from build123d import *

# Parameters (mm, degrees)
BOSS_EXTRUDE1_DEPTH = 18
SKETCH2_R           = 10
CUT_EXTRUDE1_DEPTH  = 5.6
SKETCH3_R           = 8.371578903
SKETCH3_R_2         = 6.7
BOSS_EXTRUDE2_DEPTH = 6.63


with BuildPart() as part:
    # Sketch1 → Boss-Extrude1 (new body)
    with BuildSketch(Plane.XY):
        with BuildLine():
            Line((15, 0), (75, 0))
            ThreePointArc((75, 0), (90, 15), (75, 30))
            Line((75, 30), (15, 30))
            ThreePointArc((15, 30), (0, 15), (15, 0))
        make_face()
        Polygon((15, 23.371578903), (7.75, 19.185789452), (7.75, 10.814210548), (15, 6.628421097), (22.25, 10.814210548), (22.25, 19.185789452), align=None, mode=Mode.SUBTRACT)
        Polygon((75, 23.371578903), (67.75, 19.185789452), (67.75, 10.814210548), (75, 6.628421097), (82.25, 10.814210548), (82.25, 19.185789452), align=None, mode=Mode.SUBTRACT)
    extrude(amount=BOSS_EXTRUDE1_DEPTH)

    # Sketch2 → Cut-Extrude1 (cut)
    with BuildSketch(Plane(origin=(0, 0, 0), x_dir=(-1, 0, 0), z_dir=(0, 0, -1))):
        with Locations((-75, 15)):
            Circle(SKETCH2_R)
        with Locations((-15, 15)):
            Circle(SKETCH2_R)
    extrude(amount=-CUT_EXTRUDE1_DEPTH, mode=Mode.SUBTRACT)

    # Sketch3 → Boss-Extrude2 (add)
    # profile 1 of 2: a face of its own
    with BuildSketch(Plane.XY.offset(18)):
        with Locations((75, 15)):
            Circle(SKETCH3_R)
        with Locations((75, 15)):
            Circle(SKETCH3_R_2, mode=Mode.SUBTRACT)
    # profile 2 of 2: a face of its own
    with BuildSketch(Plane.XY.offset(18)):
        with Locations((15, 15)):
            Circle(SKETCH3_R)
        with Locations((15, 15)):
            Circle(SKETCH3_R_2, mode=Mode.SUBTRACT)
    extrude(amount=-BOSS_EXTRUDE2_DEPTH)


solid = part.part
Build history of the part. All positions in model axes, mm. A direction names the side the tool comes from. Round coordinates to 2 decimals unless told otherwise and drop trailing zeros. Write each loop counter-clockwise with the first axis right and the second up, starting at its lowest first coordinate (ties: lowest second). Pieces come first, ordered by that corner, then holes. Notation, with made-up numbers: (10.5, -35.5) - (24.5, -35.5) arc R15 cw to (24.5, -6.5) - close; hole circle Ø3 at (-5.75, 55.5). An arc over 180 degrees is marked (long way). One line per question, with ' | ' between items.
1. Band-saw the part on A-A, the plane z = 7.75. Write the cut outline in (x, y), and give its area (3 significant figures).
Results are:
outline: (15, 0) - (75, 0) arc R15 ccw to (75, 30) - (15, 30) arc R15 ccw to start; hole (7.75, 10.81) - (15, 6.63) - (22.25, 10.81) - (22.25, 19.19) - (15, 23.37) - (7.75, 19.19) - close; hole (67.75, 10.81) - (75, 6.63) - (82.25, 10.81) - (82.25, 19.19) - (75, 23.37) - (67.75, 19.19) - close | area: 2,140 mm^2
2. Band-saw the part on C-C, the plane y = 20. Write the cut outline in (x, z).
Results are:
outline: (0.86, 0) - (6.34, 0) - (6.34, 5.6) - (9.16, 5.6) - (9.16, 11.37) - (10.54, 11.37) - (10.54, 18) - (0.86, 18) - close; (19.46, 11.37) - (20.84, 11.37) - (20.84, 5.6) - (23.66, 5.6) - (23.66, 0) - (66.34, 0) - (66.34, 5.6) - (69.16, 5.6) - (69.16, 11.37) - (70.54, 11.37) - (70.54, 18) - (19.46, 18) - close; (79.46, 11.37) - (80.84, 11.37) - (80.84, 5.6) - (83.66, 5.6) - (83.66, 0) - (89.14, 0) - (89.14, 18) - (79.46, 18) - close
3. Band-saw the part on D-D, the plane y = 12. Write the cut outline in (x, z), and give its area (3 significant figures).
Results are:
outline: (0.3, 0) - (5.46, 0) - (5.46, 5.6) - (7.75, 5.6) - (7.75, 11.37) - (9.01, 11.37) - (9.01, 18) - (0.3, 18) - close; (20.99, 11.37) - (22.25, 11.37) - (22.25, 5.6) - (24.54, 5.6) - (24.54, 0) - (65.46, 0) - (65.46, 5.6) - (67.75, 5.6) - (67.75, 11.37) - (69.01, 11.37) - (69.01, 18) - (20.99, 18) - close; (80.99, 11.37) - (82.25, 11.37) - (82.25, 5.6) - (84.54, 5.6) - (84.54, 0) - (89.7, 0) - (89.7, 18) - (80.99, 18) - close | area: 1,070 mm^2
4. Tool access for faces 1 (the face through (18.092, 9.056, 14.731)), 2 (the face through (7.75, 15, 8)): list every direction of +Z, -Z, +X, -X, +Y, -Y with a clear straight run to the whole face (end or side of a thin tool).
Results are:
face 1: +Z, -Z | face 2: -Z
5. Drop flat-ended pins along their axis: pin 1 Ø7 at (x, y) = (14, 17) entering from -Z; pin 2 Ø17.5 at (x, y) = (75, 15) entering from -Z; pin 3 Ø1.5 at (x, z) = (13, 3) entering from -Y. Give the stop position or say it passes through.
Results are:
pin 1: through | pin 2: z = 5.6 | pin 3: y = 0.05
6. Mould opens along Y. For faces 3 (the face through (44, 15, 18)), 4 (the face through (71.43, 21.31, 8.44)), 5 (the face through (90, 15, 9)), 6 (the face through (67.6, 14.3, 5.6)) say: released by +Y, released by -Y, zero draft, split by the parting line, or undercut.
Results are:
face 3: zero draft | face 4: undercut | face 5: split by the parting line | face 6: undercut
7. Band-saw the part on B-B, the plane x = 76.5. Write the cut outline in (y, z), and give its area (3 significant figures).
Results are:
outline: (0.08, 0) - (5.11, 0) - (5.11, 5.6) - (7.49, 5.6) - (7.49, 11.37) - (8.47, 11.37) - (8.47, 18) - (0.08, 18) - close; (21.53, 11.37) - (22.51, 11.37) - (22.51, 5.6) - (24.89, 5.6) - (24.89, 0) - (29.92, 0) - (29.92, 18) - (21.53, 18) - close | area: 253 mm^2
8. Drill centre lines: line 1 along X through (y, z) = (12.75, 5.25); line 2 along X through (y, z) = (19, 5.25); line 3 along Y through (x, z) = (75, 2.95). Where is each one in solid material? Low to high. Write a range as from..to.
Results are:
line 1: 0.17..5.26, 24.74..65.26, 84.74..89.83 | line 2: 0.54..5.83, 24.17..65.83, 84.17..89.46 | line 3: 0..5, 25..30
